Here's how the part is built. I have some questions about the finished solid (model axes, mm). Coordinates: 2 decimals unless noted, no trailing zeros. Write each loop counter-clockwise with the first axis right and the second up, starting at its lowest first coordinate (ties: lowest second). Pieces come first, ordered by that corner, then holes. Notation, with made-up numbers: (53, -9) - (107, -9) arc R16 ccw to (107, 17) - close; hole circle Ø4 at (83.25, 50.5). An arc over 180 degrees is marked (long way). Answer in a Markdown table with one row per item. Add a question column.
Item 1: If I drill on probe 1 along X at (y, z) = (-0.5, 1); probe 2 along Z at (x, y) = (-0.5, -3.55), over which ranges is the centre line in solid material (lowest first)? Write a range as from..to.
Item 2: Imagine slicing it at A-A (z = -12.5). Please give me the cut outline in (x, y).
Item 3: Imagine slicing it at D-D (x = 10). Please give me the cut outline in (y, z), plus the area to 3 significant figures.
Item 4: Imagine slicing it at C-C (y = -1.4). Please give me the cut outline in (x, z), plus the area to 3 significant figures.
Item 5: Imagine slicing it at B-B (x = -1.5). Please give me the cut outline in (y, z).
from build123d import *

# Parameters (mm, degrees)
F0_R     = 16.5
F1_DEPTH = 4
F3_DEPTH = 4.001


with BuildPart() as f1:
    # F0 (on Front) → F1 (new body)
    with BuildSketch(Plane.XZ):
        Circle(F0_R)
    extrude(amount=F1_DEPTH)

    # F2 (on face) → F3 (cut, through all)
    with BuildSketch(Plane.XZ.offset(4)):
        with BuildLine():
            ThreePointArc((-10.8181818182, -1.9917183909), (-9.5229021082, -1.3483997249), (-9, 0))
            Line((-9, 0), (-9.5, 0))
            Line((-9.5, 0), (-11, 0))
            ThreePointArc((-11, 0), (-10.9544511501, -1), (-10.8181818182, -1.9917183909))
        make_face()
        with BuildLine():
            Line((-9.5, 0), (-9, 0))
            ThreePointArc((-9, 0), (-9.5229021082, 1.3483997249), (-10.8181818182, 1.9917183909))
            ThreePointArc((-10.8181818182, 1.9917183909), (-10.9544511501, 1), (-11, 0))
            Line((-11, 0), (-9.5, 0))
        make_face()
        with BuildLine():
            ThreePointArc((0, 2), (-1.4142135624, 1.4142135624), (-2, 0))
            Line((-2, 0), (0, 0))
            Line((0, 0), (0, 2))
        make_face()
        with BuildLine():
            Line((0, 0), (-2, 0))
            ThreePointArc((-2, 0), (-1.4142135624, -1.4142135624), (0, -2))
            Line((0, -2), (0, 0))
        make_face()
        with BuildLine():
            ThreePointArc((-11, 0), (-10.9544511501, 1), (-10.8181818182, 1.9917183909))
            ThreePointArc((-10.8181818182, 1.9917183909), (-12.3483997249, 1.4770978918), (-13, 0))
            Line((-13, 0), (-11, 0))
        make_face()
        with BuildLine():
            ThreePointArc((-13, 0), (-12.3483997249, -1.4770978918), (-10.8181818182, -1.9917183909))
            ThreePointArc((-10.8181818182, -1.9917183909), (-10.9544511501, -1), (-11, 0))
            Line((-11, 0), (-13, 0))
        make_face()
        with BuildLine():
            Line((2, 0), (0, 0))
            Line((0, 0), (0, -2))
            ThreePointArc((0, -2), (1.4142135624, -1.4142135624), (2, 0))
        make_face()
        with BuildLine():
            Line((0, 2), (0, 0))
            Line((0, 0), (2, 0))
            ThreePointArc((2, 0), (1.4142135624, 1.4142135624), (0, 2))
        make_face()
        with BuildLine():
            ThreePointArc((0, 13), (-1.4770978918, 12.3483997249), (-1.9917183909, 10.8181818182))
            ThreePointArc((-1.9917183909, 10.8181818182), (-1, 10.9544511501), (0, 11))
            Line((0, 11), (0, 13))
        make_face()
        with BuildLine():
            ThreePointArc((0, 11), (-1, 10.9544511501), (-1.9917183909, 10.8181818182))
            ThreePointArc((-1.9917183909, 10.8181818182), (-1.3483997249, 9.5229021082), (0, 9))
            Line((0, 9), (0, 9.5))
            Line((0, 9.5), (0, 11))
        make_face()
        with BuildLine():
            ThreePointArc((0, -9), (-1.3483997249, -9.5229021082), (-1.9917183909, -10.8181818182))
            ThreePointArc((-1.9917183909, -10.8181818182), (-1, -10.9544511501), (0, -11))
            Line((0, -11), (0, -9.5))
            Line((0, -9.5), (0, -9))
        make_face()
        with BuildLine():
            ThreePointArc((0, -11), (-1, -10.9544511501), (-1.9917183909, -10.8181818182))
            ThreePointArc((-1.9917183909, -10.8181818182), (-1.4770978918, -12.3483997249), (0, -13))
            Line((0, -13), (0, -11))
        make_face()
        with BuildLine():
            Line((0, 9.5), (0, 9))
            ThreePointArc((0, 9), (1.3483997249, 9.5229021082), (1.9917183909, 10.8181818182))
            ThreePointArc((1.9917183909, 10.8181818182), (1, 10.9544511501), (0, 11))
            Line((0, 11), (0, 9.5))
        make_face()
        with BuildLine():
            ThreePointArc((1.9917183909, -10.8181818182), (1.3483997249, -9.5229021082), (0, -9))
            Line((0, -9), (0, -9.5))
            Line((0, -9.5), (0, -11))
            ThreePointArc((0, -11), (1, -10.9544511501), (1.9917183909, -10.8181818182))
        make_face()
        with BuildLine():
            Line((0, 13), (0, 11))
            ThreePointArc((0, 11), (1, 10.9544511501), (1.9917183909, 10.8181818182))
            ThreePointArc((1.9917183909, 10.8181818182), (1.997928525, 10.9089966535), (2, 11))
            ThreePointArc((2, 11), (1.4142135624, 12.4142135624), (0, 13))
        make_face()
        with BuildLine():
            ThreePointArc((1.9917183909, -10.8181818182), (1, -10.9544511501), (0, -11))
            Line((0, -11), (0, -13))
            ThreePointArc((0, -13), (1.4142135624, -12.4142135624), (2, -11))
            ThreePointArc((2, -11), (1.997928525, -10.9089966535), (1.9917183909, -10.8181818182))
        make_face()
        with BuildLine():
            ThreePointArc((10.8181818182, 1.9917183909), (9.5229021082, 1.3483997249), (9, 0))
            Line((9, 0), (9.5, 0))
            Line((9.5, 0), (11, 0))
            ThreePointArc((11, 0), (10.9544511501, 1), (10.8181818182, 1.9917183909))
        make_face()
        with BuildLine():
            Line((9.5, 0), (9, 0))
            ThreePointArc((9, 0), (9.5229021082, -1.3483997249), (10.8181818182, -1.9917183909))
            ThreePointArc((10.8181818182, -1.9917183909), (10.9544511501, -1), (11, 0))
            Line((11, 0), (9.5, 0))
        make_face()
        with BuildLine():
            ThreePointArc((13, 0), (12.3483997249, 1.4770978918), (10.8181818182, 1.9917183909))
            ThreePointArc((10.8181818182, 1.9917183909), (10.9544511501, 1), (11, 0))
            Line((11, 0), (13, 0))
        make_face()
        with BuildLine():
            ThreePointArc((11, 0), (10.9544511501, -1), (10.8181818182, -1.9917183909))
            ThreePointArc((10.8181818182, -1.9917183909), (12.3483997249, -1.4770978918), (13, 0))
            Line((13, 0), (11, 0))
        make_face()
    extrude(amount=-F3_DEPTH, mode=Mode.SUBTRACT)


solid = f1.part
Here are the results:
| question | item | result |
|---|---|---|
| 1 | probe 1 | x = -16.47..-12.73, -9.27..-1.73, 1.73..9.27, 12.73..16.47 |
| 1 | probe 2 | z = -16.49..-12.94, -9.06..-1.94, 1.94..9.06, 12.94..16.49 |
| 2 | outline | (-10.77, -4) - (-1.32, -4) - (-1.32, 0) - (-10.77, 0) - close; (1.32, -4) - (10.77, -4) - (10.77, 0) - (1.32, 0) - close |
| 3 | outline | (-4, -13.12) - (0, -13.12) - (0, -1.73) - (-4, -1.73) - close; (-4, 1.73) - (0, 1.73) - (0, 13.12) - (-4, 13.12) - close |
| 3 | area | 91.1 mm2 |
| 4 | outline | circle Ø33 at (0, 0); hole circle Ø4 at (-11, 0); hole circle Ø4 at (0, -11); hole circle Ø4 at (0, 0); hole circle Ø4 at (0, 11); hole circle Ø4 at (11, 0) |
| 4 | area | 792 mm2 |
| 5 | outline | (-4, -16.43) - (0, -16.43) - (0, -12.32) - (-4, -12.32) - close; (-4, -9.68) - (0, -9.68) - (0, -1.32) - (-4, -1.32) - close; (-4, 1.32) - (0, 1.32) - (0, 9.68) - (-4, 9.68) - close; (-4, 12.32) - (0, 12.32) - (0, 16.43) - (-4, 16.43) - close |
